Build history of the part. All positions in model axes, mm. A direction names the side the tool comes from. Round coordinates to 2 decimals unless told otherwise and drop trailing zeros. Loops run counter-clockwise (first coordinate to the right, second up) from the corner with the lowest first, then second, coordinate; pieces in that order, holes last. Notation, with made-up numbers: M 31.5,-17 L 66.5,-17 A4 ccw 66.5,-10 Z; hole C 46.25,45.25 d7. An arc over 180 degrees is marked long. One line per item, written item: value.
Autodesk Fusion 360 part; units mm, degrees
sketch "Sketch1" plane through (0, 0, 0) normal (0, 1, 0) x (1, 0, 0)
  line L0 (0, 0) -> (22.5, 38.9711)
  line L1 (0, 0) -> (45, 0) construction
  line L2 (22.5, 38.9711) -> (25.0981, 37.4711)
  line L3 (22.5, 38.9711) -> (25.5, 38.9711) construction
  line L4 (25.0981, 37.4711) -> (3.4641, 0)
  line L5 (25.0981, 37.4711) -> (68.366, 37.4711) construction
  line L6 (0, 0) -> (45, 0)
  line L7 (45, 0) -> (45, 3)
  line L8 (45, 3) -> (1.7321, 3)
  dimension "d1" = 45
  dimension "d2" = 60
  dimension "d3" = 30
  dimension "d4" = 3
  dimension "d5" = 120
  dimension "d6" = 45
  dimension "d7" = 3
extrude "Extrude1" add sketch "Sketch1" along normal blind 45
extrude "Extrude2" add 1 faces at (9.2321, 45, -13.9904) along direction (0, 1, 0) blind 20
fillet "Fillet1" radius 1 17 edges at (0, 32.5, 0) (22.5, 32.5, -38.9711) (11.25, 65, -19.4856) (11.25, 0, -19.4856) (22.5, 0, 0) (45, 32.5, 0) (22.5, 65, 0) (15.1471, 65, -20.2356) (25.0981, 65, -3) (15.1471, 0, -20.2356) (25.0981, 0, -3) (25.0981, 32.5, -37.4711) (23.799, 65, -38.2211) (23.799, 0, -38.2211) (45, 65, -1.5) (45, 32.5, -3) (45, 0, -1.5)
Item 1: Slice it at B-B, the plane x = 36. Give the cut face in (y, z), and give its area (3 significant figures).
Check values:
outline: M 0,-2 A1 ccw 1,-3 L 64,-3 A1 ccw 65,-2 L 65,-1 A1 ccw 64,0 L 1,0 A1 ccw 0,-1 Z
area: 194 mm2
Item 2: Pull direction Z, two halves, no side cores. Call faces 6 (the face through (10, 0, -14)), 7 (the face through (15.033, 32.059, -20.038)), 8 (the face through (23.655, 0.285, -37.957)): pulls with the +Z half, pulls with the -Z half, needs draft (parallel to the pull), parting line crosses it, or undercut.
Check values:
face 6: needs draft
face 7: undercut
face 8: pulls with the -Z half
Item 3: Which spindle directions (+Z, -Z, +X, -X, +Y, -Y) get a long thin tool onto all of the face, cutting with end or side? Do faces 1 (the face through (23, 32, 0)), 2 (the face through (25, 32, -3)), 3 (the face through (14.062, 0.285, -18.957)), 4 (the face through (14.075, 64.699, -18.949)), 5 (the face through (11.285, 32.059, -19.546)). Say none if no direction does.
Check values:
face 1: +Z, +X, -X, +Y, -Y
face 2: +X, +Y, -Y
face 3: +X, -Y
face 4: +X, +Y
face 5: -Z, -X, +Y, -Y
Item 4: Slice it at A-A, the plane y = 45.5. Give the cut face in (x, z), and give its area (3 significant figures).
Check values:
outline: M 0.87,-1.5 L 22,-38.11 A1 ccw 23.37,-38.47 L 24.23,-37.97 A1 ccw 24.6,-36.61 L 5.2,-3 L 44,-3 A1 ccw 45,-2 L 45,-1 A1 ccw 44,0 L 1.73,0 A1 ccw Z
area: 253 mm2
Item 5: Wall check: line 1 along Z through (x, y) = (40, 55.5); line 2 along X through (y, z) = (34, -1.5); line 3 along Z through (x, y) = (15.5, 20.5). Give the ranges that are in metal, low to high.
Check values:
line 1: z = -3 to 0
line 2: x = 0.87 to 45
line 3: z = -26.85 to -20.85, -3 to 0
Item 6: Drop flat-ended pins along their axis: P1, Ø1, axis at y = 24.5, z = -6.5, coming from the -X side; P2, Ø2, axis at x = 29.5, y = 54, coming from the -Z side; P3, Ø2, axis at y = 56, z = -32.5, coming from the -X side. Give the stop position or say it passes through.
Check values:
P1: stops at x = 3.46
P2: stops at z = -3
P3: stops at x = 18.19
